For this review, take the finished solid that the model builds, in its own axes (mm). Face numbers are marked on the shaded views. A direction names the side the tool comes from. Coordinates: 2 decimals unless noted, no trailing zeros. Write each loop counter-clockwise with the first axis right and the second up, starting at its lowest first coordinate (ties: lowest second). Pieces come first, ordered by that corner, then holes.
1) We need section D-D on z = -19. Write out the cut boundary in (x, y), then the cut area to 3 significant figures.
2) For the marked faces 5 and 6, list the 3-axis set-ups (+Z, -Z, +X, -X, +Y, -Y) from which the entire face can be reached by the end or side of a thin tool; tool diameter is ignored.
3) To check wall thickness, follow line 1 along X through (y, z) = (2, -14.5); line 2 along X through (y, z) = (2.75, -6); line 3 along Z through (x, y) = (-4, 2.25). State the ranges of each line that lie inside material, in increasing order.
4) Insertion check: P1, Ø2, axis at y = 2, z = -19, coming from the -X side; P2, Ø2, axis at y = 2.5, z = -17.5, coming from the -X side; P3, Ø1.2, axis at x = -8.5, y = 2, coming from the +Z side; P4, Ø2, axis at y = 3, z = -18.5, coming from the +X side. Each pin has a flat end and moves straight along its axis. Give the tip position at first contact, or say it passes through.
5) We need section C-C on y = 3.25. Write out the cut boundary in (x, z), then the cut area to 3 significant figures.
6) We need section B-B on x = -6. Write out the cut boundary in (y, z), then the cut area to 3 significant figures.
7) Mouldability with a two-part tool opening along Z and no side actions: class the marked faces 1, 2, 3 and 4 as pulls with the +Z half, pulls with the -Z half, needs draft (parallel to the pull), parting line crosses it, or undercut.
8) We need section A-A on z = -16.75. Write out the cut boundary in (x, y), then the cut area to 3 significant figures.
Autodesk Inventor part; units mm, degrees
ref_plane "YZ Plane" through (0, 0, 0) normal (1, 0, 0) x (0, 1, 0)
ref_plane "XZ Plane" through (0, 0, 0) normal (0, 1, 0) x (-1, 0, 0)
ref_plane "XY Plane" through (0, 0, 0) normal (0, 0, 1) x (1, 0, 0)
sketch "Sketch4" plane through (0, 0, 0) normal (0, 1, 0) x (-1, 0, 0)
  line L0 (0, 0) -> (12, 0)
  line L1 (12, 0) -> (12, -12)
  line L2 (12, -12) -> (9.75, -12)
  line L3 (9.75, -12) -> (9.75, -21.5)
  line L4 (9.75, -21.5) -> (2.25, -21.5)
  line L5 (2.25, -21.5) -> (2.25, -12)
  line L6 (2.25, -12) -> (0, -12)
  line L7 (0, -12) -> (0, 0)
  dimension "d17" = 12
  dimension "d18" = 12
  dimension "d19" = 7.5
  dimension "d20" = 2.25
  dimension "d21" = 9.5
extrude "Extrusion2" add sketch "Sketch4" along normal blind 6.5
sketch "Sketch5" plane through (0, 6.5, 0) normal (0, 1, 0) x (1, 0, 0)
  line L0 (-9.75, 14) -> (-7.25, 14)
  line L1 (-7.25, 14) -> (-7.25, 19.5)
  line L2 (-7.25, 19.5) -> (-9.75, 19.5)
  line L3 (-9.75, 19.5) -> (-9.75, 14)
  line L4 (-2.25, 21.5) -> (-9.75, 21.5)
  line L5 (-9.75, 21.5) -> (-9.75, 12)
  point P0 (0, 0)
  dimension "d24" = 5.5
  dimension "d25" = 2.5
  dimension "d26" = 2
extrude "Extrusion3" cut sketch "Sketch5" against normal through all
sketch "Sketch6" plane through (0, 6.5, 0) normal (0, 1, 0) x (1, 0, 0)
  circle A0 centre (-6, 6) radius 4
  line L0 (-12, 0) -> (0, 0)
  line L1 (0, 0) -> (0, 12)
  dimension "d29" = 8
  dimension "d30" = 6
  dimension "d31" = 6
extrude "Extrusion4" cut sketch "Sketch6" against normal through all
sketch "Sketch7" plane through (0, 6.5, 0) normal (0, 1, 0) x (1, 0, 0)
  line L0 (-5.25, 8.5) -> (-4.25, 8.5)
  line L1 (-4.25, 8.5) -> (-4.25, 21.5)
  line L2 (-4.25, 21.5) -> (-5.25, 21.5)
  line L3 (-5.25, 21.5) -> (-5.25, 8.5)
  line L4 (-2.25, 21.5) -> (-9.75, 21.5)
  line L5 (-2.25, 12) -> (-2.25, 21.5)
  point P0 (0, 0)
  dimension "d34" = 1
  dimension "d35" = 13
  dimension "d36" = 2
extrude "Extrusion5" cut sketch "Sketch7" against normal through all
sketch "Sketch8" plane through (-2.25, 0, -12) normal (1, 0, 0) x (0, 0, -1)
  circle A0 centre (4.75, 3.25) radius 1.65
  line L0 (0, 0) -> (9.5, 0)
  line L1 (9.5, 0) -> (9.5, 6.5)
  point P0 (-12, 0)
  dimension "d39" = 3.3
  dimension "d40" = 3.25
  dimension "d41" = 4.75
extrude "Extrusion6" cut sketch "Sketch8" against normal through all
fillet "Fillet1" radius 2 4 edges at (-12, 3.25, -12) (-12, 3.25, 0) (0, 3.25, 0) (0, 3.25, -12)
properties part number "COLLIER"
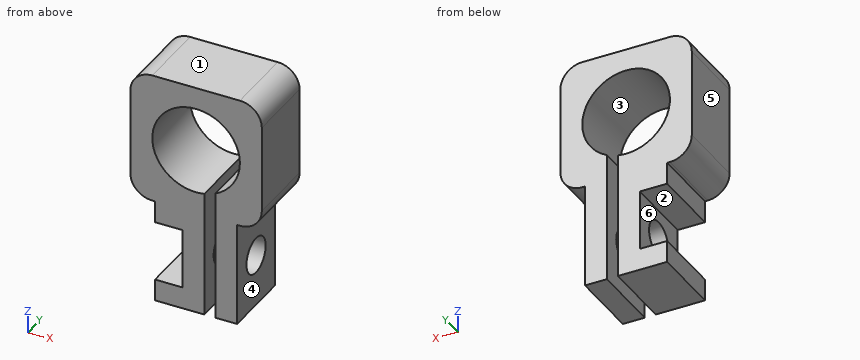
Result:
1. outline: (-7.25, 0) - (-5.25, 0) - (-5.25, 6.5) - (-7.25, 6.5) - close; (-4.25, 0) - (-2.25, 0) - (-2.25, 6.5) - (-4.25, 6.5) - close
1. area: 26.0 mm2
2. face 5: +Z, -Z, -X, +Y, -Y
2. face 6: -X, +Y, -Y
3. line 1: x = -7.25 to -5.25, -4.25 to -2.25
3. line 2: x = -12 to -10, -2 to 0
3. line 3: z = -21.5 to -18.06, -15.44 to -9.46, -2.54 to 0
4. P1: stops at x = -9.75
4. P2: stops at x = -7.25
4. P3: stops at z = 0
4. P4: stops at x = -2.25
5. outline: (-12, -10) arc R2 ccw to (-10, -12) - (-9.75, -12) - (-9.75, -14) - (-7.25, -14) - (-7.25, -15.1) - (-5.25, -15.1) - (-5.25, -9.93) arc R4 cw (long way) to (-4.25, -9.6) - (-4.25, -15.1) - (-2.25, -15.1) - (-2.25, -12) - (-2, -12) arc R2 ccw to (0, -10) - (0, -2) arc R2 ccw to (-2, 0) - (-10, 0) arc R2 ccw to (-12, -2) - close; (-9.75, -21.5) - (-5.25, -21.5) - (-5.25, -18.4) - (-7.25, -18.4) - (-7.25, -19.5) - (-9.75, -19.5) - close; (-4.25, -21.5) - (-2.25, -21.5) - (-2.25, -18.4) - (-4.25, -18.4) - close
5. area: 123 mm2
6. outline: (0, -21.5) - (6.5, -21.5) - (6.5, -10) - (0, -10) - close; (0, -2) - (6.5, -2) - (6.5, 0) - (0, 0) - close; hole circle Ø3.3 at (3.25, -16.75)
6. area: 79.2 mm2
7. face 1: pulls with the +Z half
7. face 2: undercut
7. face 3: undercut
7. face 4: needs draft
8. outline: (-7.25, 0) - (-5.25, 0) - (-5.25, 1.6) - (-7.25, 1.6) - close; (-7.25, 4.9) - (-5.25, 4.9) - (-5.25, 6.5) - (-7.25, 6.5) - close; (-4.25, 0) - (-2.25, 0) - (-2.25, 1.6) - (-4.25, 1.6) - close; (-4.25, 4.9) - (-2.25, 4.9) - (-2.25, 6.5) - (-4.25, 6.5) - close
8. area: 12.8 mm2
